```python
from build123d import *

# Parameters (mm, degrees)
SKETCH_1_W             = 56
SKETCH_1_H             = 56
SM_BASE_FLANGE_1_DEPTH = 4
SKETCH_6_R             = 24.5
SKETCH_6_R_2           = 1.6
CUT_EXTRUDE_1_DEPTH    = 4
FILLET_1_R             = 3


# Sheet-metal steps are written as plain solids
with BuildPart() as part:
    # Sketch 1 → Базовая кромка1 (new body)
    with BuildSketch(Plane.XY):
        Rectangle(SKETCH_1_W, SKETCH_1_H)
    extrude(amount=-SM_BASE_FLANGE_1_DEPTH)

    # Эскиз6 → Вырез-Вытянуть1 (cut)
    with BuildSketch(Plane.XY):
        Circle(SKETCH_6_R)
        with Locations((-24, 24)):
            Circle(SKETCH_6_R_2)
        with Locations((24, 24)):
            Circle(SKETCH_6_R_2)
        with Locations((24, -24)):
            Circle(SKETCH_6_R_2)
        with Locations((-24, -24)):
            Circle(SKETCH_6_R_2)
    extrude(amount=-CUT_EXTRUDE_1_DEPTH, mode=Mode.SUBTRACT)

    # Скругление1
    fillet_1_edges = [part.edges().sort_by_distance(p)[0] for p in [
        (28, -28, -2),
        (-28, -28, -2),
        (-28, 28, -2),
        (28, 28, -2),
    ]]
    fillet(fillet_1_edges, radius=FILLET_1_R)


solid = part.part
```
Geometry: final body of the model. Coordinates: model frame, mm. Coordinates: 2 decimals unless noted, no trailing zeros. Write each loop counter-clockwise with the first axis right and the second up, starting at its lowest first coordinate (ties: lowest second). Pieces come first, ordered by that corner, then holes. Notation, with made-up numbers: M 75,22.5 L 100,22.5 A13 cw 100,35.5 Z; hole C -36,56.5 d4. An arc over 180 degrees is marked long. Use CSV: the item, a comma, the result in double quotes. Start each with the question number.
1. Ray query, probe 1 along Y at (x, z) = (14.5, -0.4); probe 2 along Y at (x, z) = (-10, -2.6); probe 3 along X at (y, z) = (22, -2.45). Return the intervals inside material, ascending.
2. Cut plane A-A on y = 0. Return the cut outline in (x, z), plus the area to 3 significant figures.
3. Mould query, pull axis X, two halves, no side actions, for faces 1 (the face through (27.1, -27.14, -2.03)), 2 (the face through (13.17, 20.66, -1.97)), 3 (the face through (-24.208, 25.586, -1.972)), 4 (the face through (0, 28, -2)). Classes: pulls with the +X half, pulls with the -X half, needs draft (parallel to the pull), parting line crosses it, or undercut.
4. Cut plane C-C on z = -0.75. Return the cut outline in (x, y).
5. First-contact query: P1, Ø3.5, axis at x = -24, y = -24, coming from the +Z side. Flat tip, straight axial feed; report the tip coordinate or a pass-through.
Entries:
1,probe 1,"-28 to -19.75, 19.75 to 28"
1,probe 2,"-28 to -22.37, 22.37 to 28"
1,probe 3,"-28 to -10.78, 10.78 to 28"
2,outline,"M -28,-4 L -24.5,-4 L -24.5,0 L -28,0 Z; M 24.5,-4 L 28,-4 L 28,0 L 24.5,0 Z"
2,area,"28.0 mm²"
3,face 1,"pulls with the +X half"
3,face 2,"undercut"
3,face 3,"undercut"
3,face 4,"needs draft"
4,outline,"M -28,-25 A3 ccw -25,-28 L 25,-28 A3 ccw 28,-25 L 28,25 A3 ccw 25,28 L -25,28 A3 ccw -28,25 Z; hole C -24,-24 d3.2; hole C -24,24 d3.2; hole C 0,0 d49; hole C 24,-24 d3.2; hole C 24,24 d3.2"
5,P1,"z = 0"
